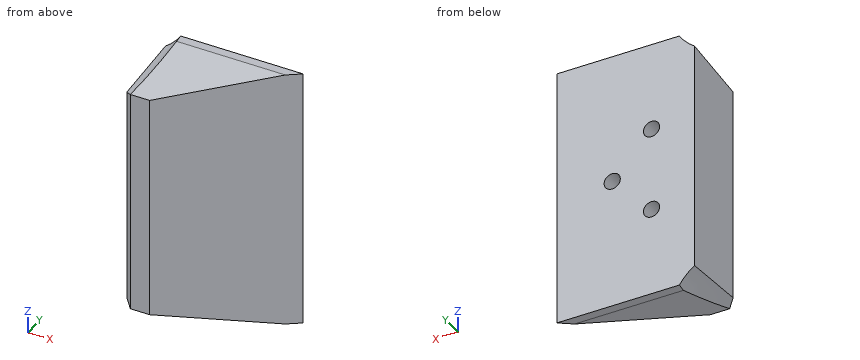
Autodesk Inventor part; units mm, degrees
ref_plane "YZ Plane" through (0, 0, 0) normal (1, 0, 0) x (0, 1, 0)
ref_plane "XZ Plane" through (0, 0, 0) normal (0, 1, 0) x (-1, 0, 0)
ref_plane "XY Plane" through (0, 0, 0) normal (0, 0, 1) x (1, 0, 0)
sketch "Sketch1" plane through (0, 0, 0) normal (0, 0, 1) x (1, 0, 0)
  line L0 (-108.119909, -0.642406) -> (-283.474909, -0.642406)
  line L1 (-142.122291, -0.642406) -> (-170.837871, -20.749272)
  line L2 (-142.122291, -0.642406) -> (-107.067041, -0.642406) construction
  line L3 (-170.837871, -20.749272) -> (-177.837871, -20.749272)
  line L4 (-177.837871, -20.749272) -> (-184.577322, -0.642406)
  line L5 (-177.837871, -20.749272) -> (-177.837871, -0.642406)
  point P0 (0, 0)
  dimension "d0" = 145
  dimension "d1" = 7
extrude "Extrusion1" add sketch "Sketch1" along normal mid plane 68.2625 contours L1 L3 L5 L0
chamfer "Chamfer1" distance 4.7625 angle 75 2 edges at (-174.3379, -20.7493, -34.1313) (-174.3379, -20.7493, 34.1313) measured on face at (-175.5045, -20.7493, -11.3771)
chamfer "Chamfer2" distance 2 angle 45 1 edges at (-177.8379, -20.7493, 0)
sketch "Sketch2" plane through (-177.837871, -0.642406, 34.13125) normal (0, 1, 0) x (1, 0, 0)
  circle A0 centre (11.158205, 23.13125) radius 2.1
  circle A1 centre (21.356244, 34.13125) radius 2.1
  circle A2 centre (11.158205, 45.13125) radius 2.1
  point P0 (177.837871, 34.13125)
extrude "Extrusion2" cut sketch "Sketch2" against normal blind 5.5
sketch "Sketch3" plane through (-177.837871, -0.642406, 34.13125) normal (0, 1, 0) x (1, 0, 0)
  ellipse E0 centre (-9.038126, 75.297581) end of major axis (-3.616987, 62.831943) minor radius 11.723829
  ellipse E1 centre (-5.030683, 77.040364) end of major axis (-0.216713, 65.970883) minor radius 10.410756
  ellipse E2 centre (-9.038126, 75.297581) end of major axis (-3.616987, 62.831943) minor radius 11.723829
  ellipse E3 centre (-5.030683, 77.040364) end of major axis (-0.216713, 65.970883) minor radius 10.410756
  circle A0 centre (-7.965707, 75.900412) radius 14.145392
  line L0 (35.71558, 68.2625) -> (35.71558, 0)
  line L1 (35.71558, 34.13125) -> (24.180949, 34.13125) construction
  circle A1 centre (-7.965707, -7.637912) radius 14.145392
  point P0 (177.837871, 34.13125)
sketch "Sketch3 outline for Extrusion3" plane through (-177.837871, -0.642406, 34.13125) normal (0, 1, 0) x (1, 0, 0)
  circle A0 centre (-7.965707, -7.637912) radius 14.145392
  circle A1 centre (-7.965707, 75.900412) radius 14.145392
extrude "Extrusion3" cut sketch "Sketch3 outline for Extrusion3" against normal blind 25.4 draft 5
properties part number "Head_Fin_Bottom"
Model file for the job. Use its own axes, mm. Coordinates: 2 decimals unless noted, no trailing zeros. Order: outer loops, then holes, each group sorted by start corner. A loop starts at its lowest first (then second) coordinate and runs counter-clockwise, first axis right, second up. Notation, with made-up numbers: (-33, 47.25) -> (-28, 47.25) arc R6 ccw to (-28, 51.25) -> close; hole circle Ø4 at (-8, -27). An arc over 180 degrees is marked (long way). Return JSON: item names as keys, results as strings. Group by question number.
Item 1: Flat gauge pins, fed straight in: P1, Ø4, axis at x = -166.68, z = 11, coming from the +Y side; P2, Ø4, axis at x = -154, z = -22.5, coming from the -Y side; P3, Ø12, axis at x = -147, y = -14.5, coming from the -Z side; P4, Ø1.5, axis at x = -159, y = -7.5, coming from the -Z side. Where does each tip first touch, or does it go through?
Item 2: Saw through at B-B on y = -8.75. Write the cut outline in (x, z).
Item 3: Saw through at D-D on x = -144.5. Write the cut outline in (y, z), then the cut area to 3 significant figures.
Item 4: Saw through at A-A on z = 11. Write the cut outline in (x, y), then the cut area to 3 significant figures.
Item 5: Wall check: line 1 along X through (y, z) = (-1.95, 11); line 2 along X through (y, z) = (-3.75, 11); line 3 along Z through (x, y) = (-156.5, -2.5). Give the ranges that are in metal, low to high. Write a range as [from, to].
Item 6: Saw through at C-C on x = -162. Write the cut outline in (y, z), then the cut area to 3 significant figures.
Values found:
{
 "1": {"P1": "stops at y = -6.14", "P2": "stops at y = -10.36", "P3": "passes through", "P4": "stops at z = -33.12"},
 "2": {"outline": "(-177.84, -29.23) arc R14.85 cw to (-174.13, -32.58) -> (-153.7, -32.58) -> (-153.7, 32.58) -> (-174.13, 32.58) arc R14.85 cw to (-177.84, 29.23) -> close"},
 "3": {"outline": "(-2.31, -34.13) -> (-0.64, -34.13) -> (-0.64, 34.13) -> (-2.31, 34.13) -> close", "area": "114 mm2"},
 "4": {"outline": "(-177.84, -18.75) -> (-175.84, -20.75) -> (-170.84, -20.75) -> (-142.12, -0.64) -> (-164.58, -0.64) -> (-164.58, -6.14) -> (-168.78, -6.14) -> (-168.78, -0.64) -> (-177.84, -0.64) -> close", "area": "404 mm2"},
 "5": {"line 1": "x = [-177.84, -168.78], [-164.58, -143.99]", "line 2": "x = [-177.84, -168.78], [-164.58, -146.56]", "line 3": "z = [-34.13, -2.1], [2.1, 34.13]"},
 "6": {"outline": "(-14.56, -31.03) -> (-2.98, -34.13) -> (-0.64, -34.13) -> (-0.64, 34.13) -> (-2.98, 34.13) -> (-14.56, 31.03) -> close", "area": "914 mm2"}
}
